Geometry: final body of the model. Coordinates: model frame, mm. A direction names the side the tool comes from. Coordinates: 2 decimals unless noted, no trailing zeros. Loops run counter-clockwise (first coordinate to the right, second up) from the corner with the lowest first, then second, coordinate; pieces in that order, holes last. Notation, with made-up numbers: (37.5, -17) - (44.5, -17) arc R18 ccw to (44.5, 13) - close; hole circle Ø10 at (60.5, 57.25). An arc over 180 degrees is marked (long way). Return JSON: item names as keys, results as strings.
from build123d import *

# Parameters (mm, degrees)
F1_DEPTH = 19.05
F2_SIZE  = 0.508
F4_DEPTH = 1.524
F6_D     = 4.3053
F6_DEPTH = 5.842
F6_TIP   = 1.2934426115


with BuildPart() as f1:
    # F0 (on Front) → F1 (new body)
    with BuildSketch(Plane.XZ):
        with BuildLine():
            Line((8.001, 0), (8.001, 19.812))
            ThreePointArc((8.001, 19.812), (-0.0717867798, 27.8126779499), (-7.9997118256, 19.6684322195))
            Line((-7.9997118256, 19.6684322195), (-7.9997118256, 0))
            Line((-7.9997118256, 0), (-0.762, 0))
            Line((-0.762, 0), (-0.762, 14.0455286734))
            ThreePointArc((-0.762, 14.0455286734), (0, 25.6286), (0.762, 14.0455286734))
            Line((0.762, 14.0455286734), (0.762, 0))
            Line((0.762, 0), (8.001, 0))
        make_face()
    extrude(amount=F1_DEPTH)

    # F2
    f2_edges = [f1.edges().sort_by_distance(p)[0] for p in [
        (0, -19.05, 25.6286),
    ]]
    chamfer(f2_edges, length=F2_SIZE)

    # F3 (on face) → F4 (cut)
    with BuildSketch(Plane.YZ.offset(8.001)):
        with BuildLine():
            Line((0, 0), (0, 11.5695536215))
            ThreePointArc((0, 11.5695536215), (-9.525, 14.986), (-19.05, 11.5695536215))
            Line((-19.05, 11.5695536215), (-19.05, 0))
            Line((-19.05, 0), (0, 0))
        make_face()
    extrude(amount=-F4_DEPTH, mode=Mode.SUBTRACT)

    # F6
    with Locations(Plane.YZ.offset(6.477)):
        with Locations((-9.525, 6.35)):
            Hole(F6_D / 2, depth=F6_DEPTH)
            with Locations((0, 0, -(F6_DEPTH + F6_TIP / 2))):  # 118° drill point
                Cone(0, F6_D / 2, F6_TIP, mode=Mode.SUBTRACT)


solid = f1.part
Item 1: Section query D-D, the plane x = 0. Return loops of the section in (y, z).
Worked out:
{"outline": "(-19.05, 26.14) - (-18.54, 25.63) - (0, 25.63) - (0, 27.81) - (-19.05, 27.81) - close"}
Item 2: First-contact query: pin 1 Ø3.5 at (y, z) = (-9.525, 6.35) entering from +X; pin 2 Ø11 at (y, z) = (-14, 7) entering from +X; pin 3 Ø7 at (x, z) = (0, 19.812) entering from +Y; pin 4 Ø5 at (x, y) = (6, -5) entering from +Z. Flat tips, straight axial feed; report the tip coordinate or a pass-through.
Worked out:
{"pin 1": "x = -0.76", "pin 2": "x = 6.48", "pin 3": "through", "pin 4": "z = 27.01"}
Item 3: Mould query, pull axis X, two halves, no side actions, for faces 5 (the face through (8.001, -9, 17)), 6 (the face through (-0.25, -18.69, 25.77)), 7 (the face through (-2, 0, 11)). Classes: +X half, -X half, draft (parallel to the pull), parting line (faces both ways), or undercut.
Worked out:
{"face 5": "+X half", "face 6": "undercut", "face 7": "draft"}
Item 4: Section query A-A, the plane z = 6.35. Return loops of the section in (x, y).
Worked out:
{"outline": "(-8, -19.05) - (-0.76, -19.05) - (-0.76, 0) - (-8, 0) - close; (0.76, -19.05) - (6.48, -19.05) - (6.48, -11.68) - (0.76, -11.68) - close; (0.76, -7.37) - (6.48, -7.37) - (6.48, 0) - (0.76, 0) - close"}
Item 5: Section query B-B, the plane z = 3.25. Return loops of the section in (x, y).
Worked out:
{"outline": "(-8, -19.05) - (-0.76, -19.05) - (-0.76, 0) - (-8, 0) - close; (0.76, -19.05) - (6.48, -19.05) - (6.48, 0) - (0.76, 0) - close"}
Item 6: Section query C-C, the plane y = -8. Return loops of the section in (x, z), and give its area (3 significant figures).
Worked out:
{"outline": "(-8, 0) - (-0.76, 0) - (-0.76, 14.05) arc R5.82 cw (long way) to (0.76, 14.05) - (0.76, 7.87) - (6.48, 7.87) - (6.48, 14.91) - (8, 14.91) - (8, 19.81) arc R8 ccw (long way) to (-8, 19.67) - close; (0.76, 0) - (6.48, 0) - (6.48, 4.83) - (0.76, 4.83) - close", "area": "250 mm^2"}
Item 7: Ray query, probe 1 along X at (y, z) = (-18, 11); probe 2 along X at (y, z) = (-10.5, 7); probe 3 along Z at (x, y) = (0, -7.5). Return the intervals inside material, ascending. Write a range as from..to.
Worked out:
{"probe 1": "-8..-0.76, 0.76..6.48", "probe 2": "-8..-0.76", "probe 3": "25.63..27.81"}
Item 8: Reachability of faces 1 (the face through (-0.762, -9, 7)), 2 (the face through (4, -9, 0)), 3 (the face through (3.58, -10.52, 4.44)), 4 (the face through (6.477, -10, 9)) from +Z, -Z, +X, -X, +Y, -Y: full face, straight path, thin tool, end or side. Return the list, or none.
Worked out:
{"face 1": "-Z, +Y, -Y", "face 2": "-Z, +X, -X, +Y, -Y", "face 3": "+X", "face 4": "-Z, +X"}
